Can you work these out from the model? Positions are in its coordinate system, mm. A direction names the side the tool comes from. Round coordinates to 2 decimals unless told otherwise and drop trailing zeros. Write each loop counter-clockwise with the first axis right and the second up, starting at its lowest first coordinate (ties: lowest second). Pieces come first, ordered by that corner, then holes. Notation, with made-up numbers: (40, 10.25) - (73, 10.25) arc R20 ccw to (73, 36.25) - close; hole circle Ø8 at (67.5, 72). An arc over 180 degrees is marked (long way). One line per item, written item: value. Start each with the question number.
(1) I want a section at A-A on z = -3.5. List the corners of the cut face in (x, y) for me, plus the area to 3 significant figures.
(2) I'm going to push flat-ended pins straight in: pin 1 Ø6.5 at (x, y) = (34, 9.5) entering from -Z; pin 2 Ø1.5 at (y, z) = (15, 8.5) entering from -X; pin 3 Ø2 at (y, z) = (6.5, 31.5) entering from -X. Where does each tip first touch, or does it pass through?
(3) On a 3-axis mill with a long thin cutter (end or side, diameter ignored), from which of +Z, -Z, +X, -X, +Y, -Y can I reach the whole of each face in a straight line? I mean faces 1 (the face through (32.89, 1.54, -13.96)), 2 (the face through (-30, 10, -5)), 3 (the face through (5, 20, 30)). Say none if no direction works.
(4) I want a section at C-C on x = -34. List the corners of the cut face in (y, z) for me, plus the area to 3 significant figures.
(5) I want a section at B-B on y = 18. List the corners of the cut face in (x, z) for me, plus the area to 3 significant figures.
(6) I want a section at D-D on x = -21. List the corners of the cut face in (y, z) for me, plus the area to 3 significant figures.
(7) Thinking about a two-plate mould opening in Y: for faces 4 (the face through (34, 18, -17)), 5 (the face through (34, 10, -11)), 6 (the face through (-34, 10, -11)), 7 (the face through (5, 0, 30)), which applies, +Y half, -Y half, draft (parallel to the pull), parting line (faces both ways), or undercut?
(8) If I drill on L1, parallel to X at y = 3, z = 0.5; L2, parallel to X at y = 14.5, z = 5.5; L3, parallel to Z at x = 16, y = 2, over which ranges is the centre line in solid material (lowest first)? Write a range as from..to.
from build123d import *

# Parameters (mm, degrees)
EXTRUDE_1_DEPTH = 20
SKETCH_3_R      = 1.2
EXTRUDE_2_DEPTH = 6


with BuildPart() as part:
    # 草图2 → 凸台-拉伸1 (new body)
    with BuildSketch(Plane(origin=(0, 0, 0), x_dir=(1, 0, 0), z_dir=(0, 1, 0))):
        with BuildLine():
            Line((-30, 0), (-30, 11))
            Line((-30, 11), (-38, 11))
            Line((-38, 11), (-38, 0))
            ThreePointArc((-38, 0), (0, -38), (38, 0))
            Line((38, 0), (38, 11))
            Line((38, 11), (30, 11))
            Line((30, 11), (30, 0))
            ThreePointArc((30, 0), (0, -30), (-30, 0))
        make_face()
    extrude(amount=EXTRUDE_1_DEPTH)

    # 草图3 → 凸台-拉伸2 (add)
    with BuildSketch(Plane(origin=(0, 0, -11), x_dir=(-1, 0, 0), z_dir=(0, 0, -1))):
        with Locations((-34, 18)):
            Circle(SKETCH_3_R)
        with Locations((-34, 2)):
            Circle(SKETCH_3_R)
        with Locations((34, 18)):
            Circle(SKETCH_3_R)
        with Locations((34, 2)):
            Circle(SKETCH_3_R)
    extrude(amount=EXTRUDE_2_DEPTH)


solid = part.part
Established:
1. outline: (-38, 0) - (-30, 0) - (-30, 20) - (-38, 20) - close; (30, 0) - (38, 0) - (38, 20) - (30, 20) - close
1. area: 320 mm2
2. pin 1: z = -11
2. pin 2: x = -37.2
2. pin 3: x = -22.67
3. face 1: -Z
3. face 2: -Z, +Y, -Y
3. face 3: +Z, -Z, +X, -X, +Y
4. outline: (0, -11) - (0.8, -11) - (0.8, -17) - (3.2, -17) - (3.2, -11) - (16.8, -11) - (16.8, -17) - (19.2, -17) - (19.2, -11) - (20, -11) - (20, 16.97) - (0, 16.97) - close
4. area: 588 mm2
5. outline: (-38, -11) - (-35.2, -11) - (-35.2, -17) - (-32.8, -17) - (-32.8, -11) - (-30, -11) - (-30, 0) arc R30 cw to (30, 0) - (30, -11) - (32.8, -11) - (32.8, -17) - (35.2, -17) - (35.2, -11) - (38, -11) - (38, 0) arc R38 ccw to (-38, 0) - close
5. area: 1,060 mm2
6. outline: (0, 21.42) - (20, 21.42) - (20, 31.67) - (0, 31.67) - close
6. area: 205 mm2
7. face 4: draft
7. face 5: undercut
7. face 6: undercut
7. face 7: -Y half
8. L1: -38..-30, 30..38
8. L2: -37.6..-29.49, 29.49..37.6
8. L3: 25.38..34.47
